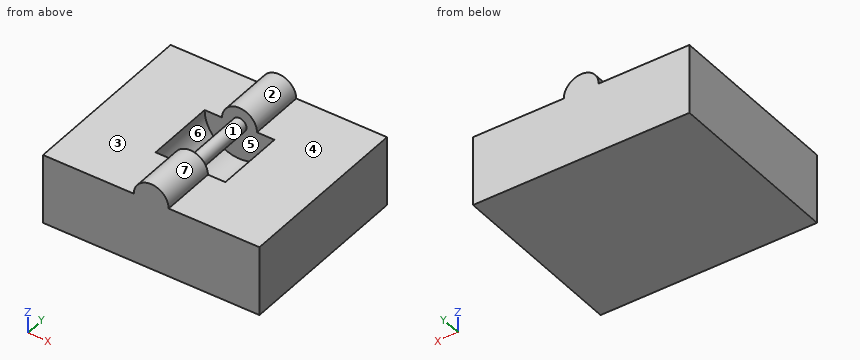
from build123d import *

# Parameters (mm, degrees)
F0_W     = 31
F0_H     = 10
F1_DEPTH = 13
F2_R     = 1
F3_DEPTH = 20
F4_R     = 2.5
F5_DEPTH = 10
F6_R     = 2.5
F7_DEPTH = 10
F8_R     = 5
F8_R_2   = 1
F9_DEPTH = 5


with BuildPart() as f1:
    # F0 (on Front) → F1 (new body, symmetric)
    with BuildSketch(Plane.XZ):
        with Locations((15.5, 5)):
            Rectangle(F0_W, F0_H)
    extrude(amount=F1_DEPTH, both=True)

    # F2 (on face) → F3 (join)
    with BuildSketch(Plane.XZ.offset(13)):
        with Locations((15.5, 10)):
            Circle(F2_R)
    extrude(amount=-F3_DEPTH)

    # F4 (on face) → F5 (join)
    with BuildSketch(Plane.XZ.offset(13)):
        with Locations((15.5, 10)):
            Circle(F4_R)
    extrude(amount=-F5_DEPTH)

    # F6 (on face) → F7 (join)
    with BuildSketch(Plane(origin=(0, 13, 0), x_dir=(-1, 0, 0), z_dir=(0, 1, 0))):
        with Locations((-15.5, 10)):
            Circle(F6_R)
    extrude(amount=-F7_DEPTH)

    # F8 (on Front) → F9 (cut, symmetric)
    with BuildSketch(Plane.XZ):
        with Locations((15.5, 10)):
            Circle(F8_R)
        with Locations((15.5, 10)):
            Circle(F8_R_2, mode=Mode.SUBTRACT)
    extrude(amount=F9_DEPTH, both=True, mode=Mode.SUBTRACT)


solid = f1.part
Geometry check sheet. Reference: the model listing, model coordinates, mm. Face numbers are marked on the shaded views. A direction names the side the tool comes from. Round coordinates to 2 decimals unless told otherwise and drop trailing zeros. Loops run counter-clockwise (first coordinate to the right, second up) from the corner with the lowest first, then second, coordinate; pieces in that order, holes last. Notation, with made-up numbers: (82, -28.5) - (113, -28.5) arc R22 ccw to (113, -14.5) - close; hole circle Ø7 at (11.5, 70.25). An arc over 180 degrees is marked (long way). One line per question, with ' | ' between items. Start each with the question number.
1. Cross-section at B-B on z = 11.5. Record the cut outline in (x, y), then the cut area to 3 significant figures.
2. Cross-section at A-A on y = -0.5. Record the cut outline in (x, z).
3. Scan lines: line 1 (Y direction, x = 18, z = 6.25); line 2 (Z direction, x = 22.5, y = 7); line 3 (X direction, y = 1.75, z = 8.5). Record each from-to range of solid material in increasing order. Write a range as [from, to].
4. Cross-section at D-D on z = 9.5. Record the cut outline in (x, y), then the cut area to 3 significant figures.
5. Cross-section at C-C on x = 15.5. Record the cut outline in (y, z), then the cut area to 3 significant figures.
6. Tool access check on the marked faces 1, 2 and 3. Record the directions out of +Z, -Z, +X, -X, +Y, -Y that give a thin tool (end or side, any length) a straight path to the whole face; none if there is none.
7. Draft check along X on the marked faces 4, 5, 6 and 7. Enter one of: released by +X, released by -X, zero draft, split by the parting line, or undercut.
8. Depth check by flat-ended pin: pin 1 (4 mm diameter, centred on x = 9, y = -6, fed in from +Z). Enter the tip coordinate at first touch or a pass-through.
Taken from the geometry:
1) outline: (13.5, -13) - (17.5, -13) - (17.5, -5) - (13.5, -5) - close; (13.5, 5) - (17.5, 5) - (17.5, 13) - (13.5, 13) - close | area: 64.0 mm²
2) outline: (0, 0) - (31, 0) - (31, 10) - (20.5, 10) arc R5 cw to (10.5, 10) - (0, 10) - close; circle Ø2 at (15.5, 10)
3) line 1: [-13, -5], [5, 13] | line 2: [0, 10] | line 3: [0, 10.73], [20.27, 31]
4) outline: (0, -13) - (31, -13) - (31, 13) - (0, 13) - close; hole (10.53, -5) - (14.63, -5) - (14.63, 5) - (10.53, 5) - close; hole (16.37, -5) - (20.47, -5) - (20.47, 5) - (16.37, 5) - close | area: 724 mm²
5) outline: (-13, 0) - (13, 0) - (13, 12.5) - (5, 12.5) - (5, 11) - (-5, 11) - (-5, 12.5) - (-13, 12.5) - close; hole (-5, 5) - (5, 5) - (5, 9) - (-5, 9) - close | area: 270 mm²
6) face 1: none | face 2: +Z, +Y, -Y | face 3: +Z, -X, +Y, -Y
7) face 4: zero draft | face 5: undercut | face 6: undercut | face 7: split by the parting line
8) pin 1: z = 10
